Autodesk Inventor part; units mm, degrees
ref_plane "YZ Plane" through (0, 0, 0) normal (1, 0, 0) x (0, 1, 0)
ref_plane "XZ Plane" through (0, 0, 0) normal (0, 1, 0) x (-1, 0, 0)
ref_plane "XY Plane" through (0, 0, 0) normal (0, 0, 1) x (1, 0, 0)
sketch "Sketch1" plane through (0, 0, 0) normal (0, 1, 0) x (-1, 0, 0)
  circle A0 centre (0, 0) radius 9
  circle A1 centre (0, 0) radius 2.5
  circle A2 centre (7, 0) radius 1.2
  circle A3 centre (0, 7) radius 1.2
  circle A4 centre (-7, 0) radius 1.2
  circle A5 centre (0, -7) radius 1.2
  dimension "d0" = 18
  dimension "d1" = 5
  dimension "d2" = 2.4
  dimension "d3" = 7
  dimension "d6" = 360
extrude "Extrusion1" add sketch "Sketch1" along normal blind 5
properties part number "Motor_adaptor"
The model under review builds one solid part; all positions refer to its coordinate system, in mm. Round coordinates to 2 decimals unless told otherwise and drop trailing zeros. Loops run counter-clockwise (first coordinate to the right, second up) from the corner with the lowest first, then second, coordinate; pieces in that order, holes last. Notation, with made-up numbers: (39.5, 6) - (85.5, 6) arc R21 ccw to (85.5, 35) - close; hole circle Ø1 at (35.5, 86). An arc over 180 degrees is marked (long way). Use CSV: the item, a comma, the result in double quotes.
(1) Clearance check with flat-ended pins moving along their axes: P1, Ø3, axis at y = 3, z = -5.5, coming from the -X side; P2, Ø2, axis at x = -2, y = 4.5, coming from the -Z side. State where each tip first meets the part, or that it passes through.
Working result:
P1,"stops at x = -8.06"
P2,"stops at z = -8.94"
(2) Take a section at D-D, the plane x = 7. Give the boundary of the cut face in (y, z), plus the area to 3 significant figures.
Working result:
outline,"(0, -5.66) - (5, -5.66) - (5, -1.2) - (0, -1.2) - close; (0, 1.2) - (5, 1.2) - (5, 5.66) - (0, 5.66) - close"
area,"44.6 mm^2"
(3) Take a section at A-A, the plane z = 0. Give the boundary of the cut face in (x, y).
Working result:
outline,"(-9, 0) - (-8.2, 0) - (-8.2, 5) - (-9, 5) - close; (-5.8, 0) - (-2.5, 0) - (-2.5, 5) - (-5.8, 5) - close; (2.5, 0) - (5.8, 0) - (5.8, 5) - (2.5, 5) - close; (8.2, 0) - (9, 0) - (9, 5) - (8.2, 5) - close"
(4) Take a section at C-C, the plane y = 4.15. Give the boundary of the cut face in (x, z), plus the area to 3 significant figures.
Working result:
outline,"circle Ø18 at (0, 0); hole circle Ø2.4 at (-7, 0); hole circle Ø5 at (0, 0); hole circle Ø2.4 at (0, -7); hole circle Ø2.4 at (0, 7); hole circle Ø2.4 at (7, 0)"
area,"217 mm^2"
(5) For line 1 (Z direction, x = 0, y = 1.7); line 2 (Z direction, x = 0.75, y = 1); line 3 (X direction, y = 1.9, z = 2), list the stretches that pass through material, from the lowest coordinate up.
Working result:
line 1,"z = -9 to -8.2, -5.8 to -2.5, 2.5 to 5.8, 8.2 to 9"
line 2,"z = -8.97 to -7.94, -6.06 to -2.38, 2.38 to 6.06, 7.94 to 8.97"
line 3,"x = -8.77 to -1.5, 1.5 to 8.77"
(6) The part is to be moulded in two halves that separate along X. For faces 1 (the cylindrical face through (1.172, 2.465, -8.923)), 2 (the flat face through (-2, 0, -2)), 3 (the cylindrical face through (8.2, 2.46, -0.05)), say which applies: pulls with the +X half, pulls with the -X half, needs draft (parallel to the pull), parting line crosses it, or undercut.
Working result:
face 1,"parting line crosses it"
face 2,"needs draft"
face 3,"undercut"
(7) Take a section at B-B, the plane x = 0. Give the boundary of the cut face in (y, z), plus the area to 3 significant figures.
Working result:
outline,"(0, -9) - (5, -9) - (5, -8.2) - (0, -8.2) - close; (0, -5.8) - (5, -5.8) - (5, -2.5) - (0, -2.5) - close; (0, 2.5) - (5, 2.5) - (5, 5.8) - (0, 5.8) - close; (0, 8.2) - (5, 8.2) - (5, 9) - (0, 9) - close"
area,"41.0 mm^2"
